Read the model definition and answer for the solid it produces. Units are mm, in the model's axes. Face numbers are marked on the shaded views. A direction names the side the tool comes from. Coordinates: 2 decimals unless noted, no trailing zeros. Order: outer loops, then holes, each group sorted by start corner. A loop starts at its lowest first (then second) coordinate and runs counter-clockwise, first axis right, second up. Notation, with made-up numbers: M 13.5,44.5 L 28.5,44.5 A24 ccw 28.5,80.5 Z; hole C 40.5,-12.5 d3. An arc over 180 degrees is marked long. Use a Markdown table: item, result. Add a question column.
1) Find section D-D on z = 0.4. Write down the section's boundary in (x, y) (3 decimals).
2) The mould has two halves that part along X. Classify the marked faces 1, 2 and 3: released by +X, released by -X, zero draft, split by the parting line, or undercut.
3) For the marked faces 4 and 5, determine the directions among +Z, -Z, +X, -X, +Y, -Y from which every point of the face is accessible in a straight line to the end or side of a thin tool.
4) Find section C-C on z = 3.4. Write down the section's boundary in (x, y).
5) Find section B-B on x = -15.25. Write down the section's boundary in (y, z).
6) Find section A-A on y = 3.75. Write down the section's boundary in (x, z), plus the area to 3 significant figures.
7) Each of these flat-tipped pins is pushed along its axis until it touches: pin 1 Ø1.5 at (x, z) = (-16, -0.5) entering from -Y; pin 2 Ø0.9 at (y, z) = (0, 1.5) entering from -X; pin 3 Ø1.5 at (x, y) = (-12.5, 5) entering from +Z; pin 4 Ø2 at (x, z) = (-4, 3.5) entering from -Y. Where does it stop, or does it pass through?
8) Find the intervals of material crossed by probe 1 along Y at (x, z) = (-15.25, 1.5); probe 2 along Z at (x, y) = (-5, -4.75); probe 3 along Y at (x, z) = (-15.25, 2.45), in increasing order. Write a range as [from, to].
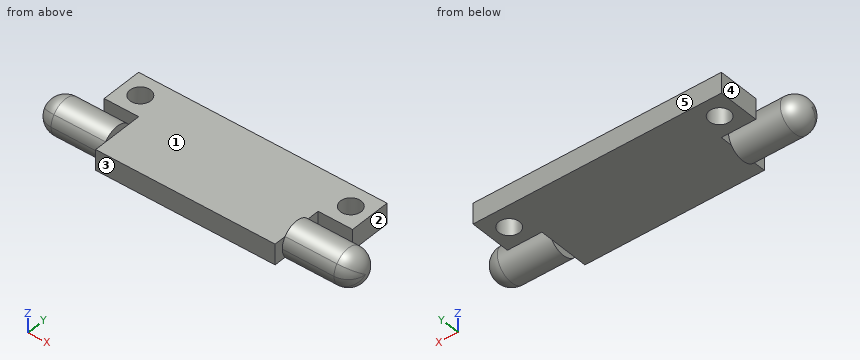
from build123d import *

# Parameters (mm, degrees)
F0_R     = 1.5
F1_DEPTH = 3
F3_DEPTH = 10
F4_R     = 2.5


# Not quite as in the source:
# - a pattern or mirror of a feature is missing from the dataset's text; its kind, count and spacing are read off the source's solid


with BuildPart() as f1:
    # F0 (on Top) → F1 (new body)
    with BuildSketch(Plane.XY):
        Polygon((18, 0.75), (18, 6.75), (-18, 6.75), (-18, 0.75), (-13, 0.75), (-13, -6.75), (13, -6.75), (13, 0.75), align=None)
        with Locations((-15.25, 3.75)):
            Circle(F0_R, mode=Mode.SUBTRACT)
        with Locations((15.25, 3.75)):
            Circle(F0_R, mode=Mode.SUBTRACT)
    extrude(amount=F1_DEPTH)

    # F2 (on face) → F3 (join)
    with BuildSketch(Plane(origin=(-13, 0, 0), x_dir=(0, -1, 0), z_dir=(-1, 0, 0))):
        with BuildLine():
            ThreePointArc((1, 0), (3, -1), (5, 0))
            Line((5, 0), (1, 0))
        make_face()
        with BuildLine():
            ThreePointArc((5, 0), (5.3717082451, 0.709430585), (5.5, 1.5))
            ThreePointArc((5.5, 1.5), (5.3717082451, 2.290569415), (5, 3))
            Line((5, 3), (1, 3))
            ThreePointArc((1, 3), (0.5, 1.5), (1, 0))
            Line((1, 0), (5, 0))
        make_face()
        with BuildLine():
            Line((1, 3), (5, 3))
            ThreePointArc((5, 3), (3, 4), (1, 3))
        make_face()
    f3 = extrude(amount=F3_DEPTH)

    # F3_copies: F3 across plane
    add(f3.mirror(Plane(origin=(0, 0, 0), x_dir=(0, 0, 1), z_dir=(1, 0, 0))))

    # F4
    f4_edges = [f1.edges().sort_by_distance(p)[0] for p in [
        (-23, -1, 0),
        (23, -1, 0),
    ]]
    fillet(f4_edges, radius=F4_R)


solid = f1.part
Check result:
| question | item | result |
|---|---|---|
| 1 | outline | M -20.5,-5.245 L -13,-5.245 L -13,-6.75 L 13,-6.75 L 13,-5.245 L 20.5,-5.245 A2.245 ccw 20.5,-0.755 L 13,-0.755 L 13,0.75 L 18,0.75 L 18,6.75 L -18,6.75 L -18,0.75 L -13,0.75 L -13,-0.755 L -20.5,-0.755 A2.245 ccw Z; hole C -15.25,3.75 d3; hole C 15.25,3.75 d3 |
| 2 | face 1 | undercut |
| 2 | face 2 | released by +X |
| 2 | face 3 | zero draft |
| 3 | face 4 | +Z, -Z, -X, +Y |
| 3 | face 5 | +Z, -Z, +X, -X, +Y |
| 4 | outline | M -20.5,-4.62 L -13,-4.62 L -13,-1.38 L -20.5,-1.38 A1.62 ccw Z; M 13,-4.62 L 20.5,-4.62 A1.62 ccw 20.5,-1.38 L 13,-1.38 Z |
| 5 | outline | C -3,1.5 d5; M 0.75,0 L 2.25,0 L 2.25,3 L 0.75,3 Z; M 5.25,0 L 6.75,0 L 6.75,3 L 5.25,3 Z |
| 6 | outline | M -18,0 L -16.75,0 L -16.75,3 L -18,3 Z; M -13.75,0 L 13.75,0 L 13.75,3 L -13.75,3 Z; M 16.75,0 L 18,0 L 18,3 L 16.75,3 Z |
| 6 | area | 90.0 mm2 |
| 7 | pin 1 | stops at y = -5.17 |
| 7 | pin 2 | stops at x = -13 |
| 7 | pin 3 | stops at z = 3 |
| 7 | pin 4 | stops at y = -6.75 |
| 8 | probe 1 | y = [-5.5, -0.5], [0.75, 2.25], [5.25, 6.75] |
| 8 | probe 2 | z = [0, 3] |
| 8 | probe 3 | y = [-5.31, -0.69], [0.75, 2.25], [5.25, 6.75] |
